Can you work these out from the model? Positions are in its coordinate system, mm. Face numbers are marked on the shaded views. A direction names the side the tool comes from. Give positions to 0.01 mm unless a question says otherwise; leave off trailing zeros. Order: outer loops, then holes, each group sorted by start corner. A loop starts at its lowest first (then second) coordinate and runs counter-clockwise, first axis right, second up. Notation, with made-up numbers: (60.5, 37.5) - (113.5, 37.5) arc R22 ccw to (113.5, 76.5) - close; hole circle Ø3 at (23, -3). An arc over 180 degrees is marked (long way). Use one line per item in the form item = value. Start each with the question number.
1) Suppose I cut it at B-B, the plane x = -105. Write out the boundary of the cut face in (y, z).
2) Please list where these lines run through material, in increasing order: probe 1 along Y at (x, z) = (-10, 1); probe 2 along Y at (x, z) = (-25, 1.2); probe 3 along Y at (x, z) = (-105, 1).
3) We'd pull the mould along Y, two halves only. Please class the marked faces 1, 2 and 3: released by +Y, released by -Y, zero draft, split by the parting line, or undercut.
4) Suppose I cut it at A-A, the plane y = 55. Write out the boundary of the cut face in (x, z).
5) For pin 1 (9.5 mm diameter, centred on x = -10, y = 40, fed in from +Z); pin 2 (3 mm diameter, centred on y = 57, z = -14.5, fed in from +X); pin 3 (5 mm diameter, centred on x = -96.5, y = 41, fed in from -Z), each with a flat end and sliding along its axis, tell me the tip position at first contact or that it passes through.
6) Suppose I cut it at D-D, the plane x = -25. Write out the boundary of the cut face in (y, z).
7) Suppose I cut it at C-C, the plane z = -10. Write out the boundary of the cut face in (x, y), and give its area (3 significant figures).
8) Which directions (+Z, -Z, +X, -X, +Y, -Y) give clear straight access to the entire face, cutting with the end or side of a thin tool? Please do the marked faces 4 and 5.
```python
from build123d import *

# Parameters (mm, degrees)
SKETCH_W      = 115
SKETCH_H      = 65
SKETCH_R      = 6
PAD_DEPTH     = 2
SKETCH001_W   = 115
SKETCH001_H   = 65
SKETCH001_W_2 = 111
SKETCH001_H_2 = 61
PAD001_DEPTH  = 65
SKETCH002_R   = 6
POCKET_DEPTH  = 2


with BuildPart() as part:
    # Sketch → Pad (new body)
    with BuildSketch(Plane.XY):
        with Locations((-57.5, 32.5)):
            Rectangle(SKETCH_W, SKETCH_H)
        with Locations((-10, 25)):
            Circle(SKETCH_R, mode=Mode.SUBTRACT)
        with Locations((-10, 10)):
            Circle(SKETCH_R, mode=Mode.SUBTRACT)
        with Locations((-10, 40)):
            Circle(SKETCH_R, mode=Mode.SUBTRACT)
        with Locations((-10, 55)):
            Circle(SKETCH_R, mode=Mode.SUBTRACT)
        with Locations((-25, 25)):
            Circle(SKETCH_R, mode=Mode.SUBTRACT)
        with Locations((-25, 40)):
            Circle(SKETCH_R, mode=Mode.SUBTRACT)
        with Locations((-25, 10)):
            Circle(SKETCH_R, mode=Mode.SUBTRACT)
        with Locations((-50, 10)):
            Circle(SKETCH_R, mode=Mode.SUBTRACT)
        with Locations((-50, 25)):
            Circle(SKETCH_R, mode=Mode.SUBTRACT)
        with Locations((-50, 40)):
            Circle(SKETCH_R, mode=Mode.SUBTRACT)
        with Locations((-50, 55)):
            Circle(SKETCH_R, mode=Mode.SUBTRACT)
        with Locations((-65, 40)):
            Circle(SKETCH_R, mode=Mode.SUBTRACT)
        with Locations((-65, 25)):
            Circle(SKETCH_R, mode=Mode.SUBTRACT)
        with Locations((-65, 10)):
            Circle(SKETCH_R, mode=Mode.SUBTRACT)
        with Locations((-90, 55)):
            Circle(SKETCH_R, mode=Mode.SUBTRACT)
        with Locations((-90, 40)):
            Circle(SKETCH_R, mode=Mode.SUBTRACT)
        with Locations((-90, 25)):
            Circle(SKETCH_R, mode=Mode.SUBTRACT)
        with Locations((-90, 10)):
            Circle(SKETCH_R, mode=Mode.SUBTRACT)
        with Locations((-105, 10)):
            Circle(SKETCH_R, mode=Mode.SUBTRACT)
        with Locations((-105, 25)):
            Circle(SKETCH_R, mode=Mode.SUBTRACT)
    extrude(amount=PAD_DEPTH)

    # Sketch001 (on Face25 of Pad) → Pad001 (join)
    with BuildSketch(Plane(origin=(0, 0, 0), x_dir=(1, 0, 0), z_dir=(0, 0, -1))):
        with Locations((-57.5, -32.5)):
            Rectangle(SKETCH001_W, SKETCH001_H)
        with Locations((-57.5, -32.5)):
            Rectangle(SKETCH001_W_2, SKETCH001_H_2, mode=Mode.SUBTRACT)
    extrude(amount=PAD001_DEPTH)

    # Sketch002 (on Face28 of Pad001) → Pocket (cut)
    with BuildSketch(Plane.XZ):
        with Locations((-57.5, -65)):
            Circle(SKETCH002_R)
    extrude(amount=-POCKET_DEPTH, mode=Mode.SUBTRACT)


solid = part.part
```
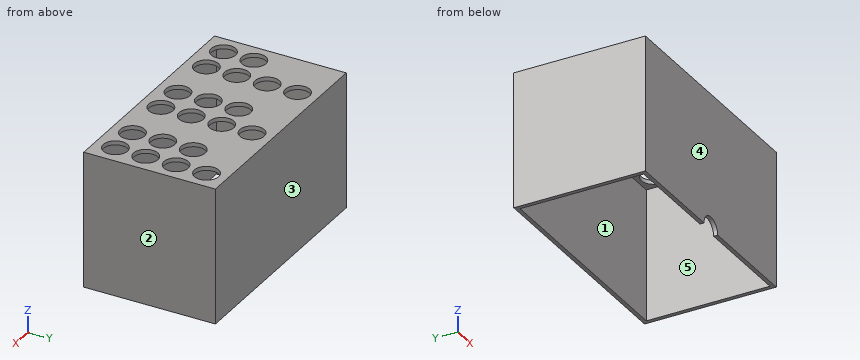
Result sheet:
q1.outline = (0, -65) - (2, -65) - (2, 0) - (4, 0) - (4, 2) - (0, 2) - close; (16, 0) - (19, 0) - (19, 2) - (16, 2) - close; (31, 0) - (63, 0) - (63, -65) - (65, -65) - (65, 2) - (31, 2) - close
q2.probe_1 = 0 to 4, 16 to 19, 31 to 34, 46 to 49, 61 to 65
q2.probe_2 = 0 to 4, 16 to 19, 31 to 34, 46 to 65
q2.probe_3 = 0 to 4, 16 to 19, 31 to 65
q3.face_1 = undercut
q3.face_2 = zero draft
q3.face_3 = released by +Y
q4.outline = (-115, -65) - (-113, -65) - (-113, 0) - (-96, 0) - (-96, 2) - (-115, 2) - close; (-84, 0) - (-56, 0) - (-56, 2) - (-84, 2) - close; (-44, 0) - (-16, 0) - (-16, 2) - (-44, 2) - close; (-4, 0) - (-2, 0) - (-2, -65) - (0, -65) - (0, 2) - (-4, 2) - close
q5.pin_1 = through
q5.pin_2 = 0
q5.pin_3 = 0
q6.outline = (0, -65) - (2, -65) - (2, 0) - (4, 0) - (4, 2) - (0, 2) - close; (16, 0) - (19, 0) - (19, 2) - (16, 2) - close; (31, 0) - (34, 0) - (34, 2) - (31, 2) - close; (46, 0) - (63, 0) - (63, -65) - (65, -65) - (65, 2) - (46, 2) - close
q7.outline = (-115, 0) - (0, 0) - (0, 65) - (-115, 65) - close; hole (-113, 2) - (-2, 2) - (-2, 63) - (-113, 63) - close
q7.area = 704 mm²
q8.face_4 = +Z, -Z, +X, -X, -Y
q8.face_5 = -Z
